Check sheet for the drawn part. Datum: minimum x, y, z corner. Units: mm. Round coordinates to 2 decimals unless told otherwise and drop trailing zeros. Write each loop counter-clockwise with the first axis right and the second up, starting at its lowest first coordinate (ties: lowest second). Pieces come first, ordered by that corner, then holes. Notation, with made-up numbers: (53, 35) - (63, 35) arc R22 ccw to (63, 47) - close; hole circle Ø5 at (54.25, 81). An arc over 180 degrees is marked (long way). Answer as a JSON object with one key per item and string values. Group by question number.
1) Go/stop test with flat-tipped pins: pin 1 Ø1.5 at (x, y) = (11, 2) entering from +Z; pin 2 Ø1.5 at (y, z) = (2, 32) entering from +X; pin 3 Ø0.9 at (y, z) = (1.5, 30) entering from -X. Record where each tip stops, or that it passes through.
2) Section check C-C (y = 2.35). Enter the section's corners in (x, z).
3) Thickness scan on line 1 (Z direction, x = 10, y = 2.2); line 2 (X direction, y = 2.3, z = 6.5); line 3 (X direction, y = 1.75, z = 34). Record the ranges inside material, lowest first.
4) Section check A-A (z = 31.5). Enter the section's corners in (x, y), then the cut area to 3 significant figures.
5) Section check B-B (x = 10). Enter the section's corners in (y, z), then the cut area to 3 significant figures.
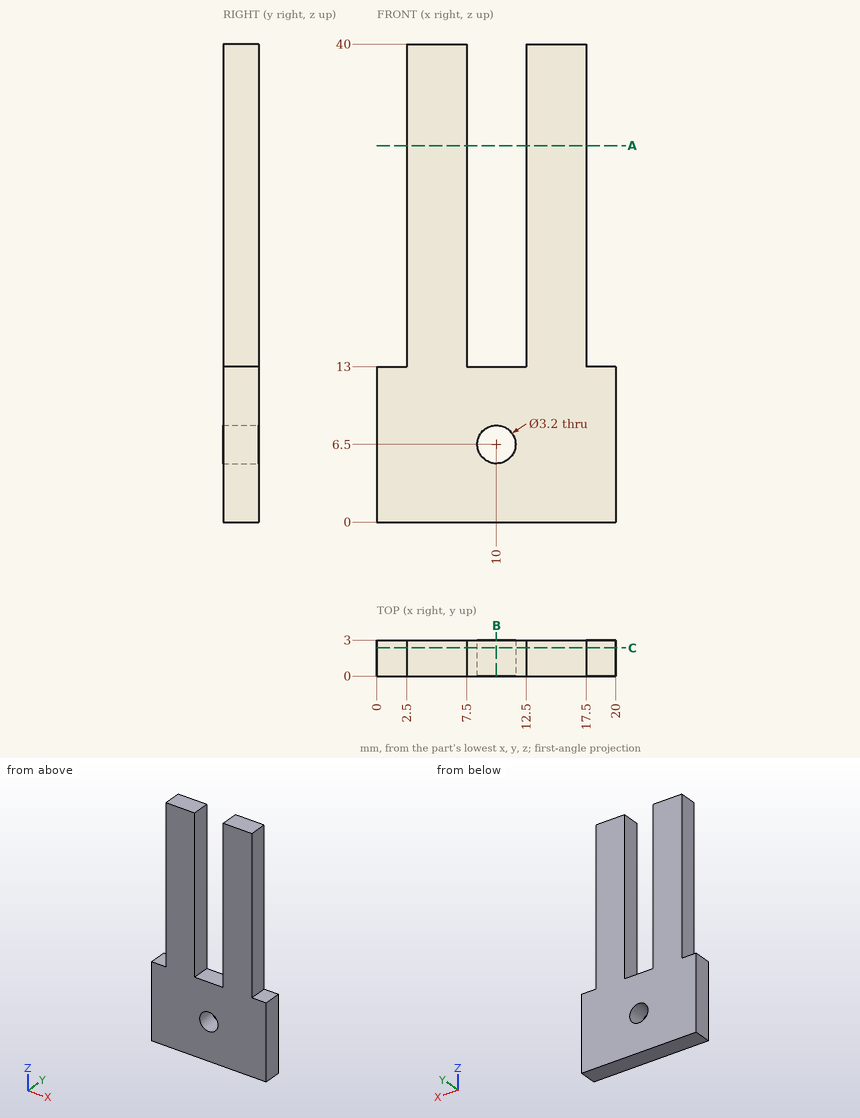
Returned:
{
 "1": {"pin 1": "z = 13", "pin 2": "x = 17.5", "pin 3": "x = 2.5"},
 "2": {"outline": "(0, 0) - (20, 0) - (20, 13) - (17.5, 13) - (17.5, 40) - (12.5, 40) - (12.5, 13) - (7.5, 13) - (7.5, 40) - (2.5, 40) - (2.5, 13) - (0, 13) - close; hole circle Ø3.2 at (10, 6.5)"},
 "3": {"line 1": "0 to 4.9, 8.1 to 13", "line 2": "0 to 8.4, 11.6 to 20", "line 3": "2.5 to 7.5, 12.5 to 17.5"},
 "4": {"outline": "(2.5, 0) - (7.5, 0) - (7.5, 3) - (2.5, 3) - close; (12.5, 0) - (17.5, 0) - (17.5, 3) - (12.5, 3) - close", "area": "30.0 mm2"},
 "5": {"outline": "(0, 0) - (3, 0) - (3, 4.9) - (0, 4.9) - close; (0, 8.1) - (3, 8.1) - (3, 13) - (0, 13) - close", "area": "29.4 mm2"}
}
